```python
from build123d import *

# Parameters (mm, degrees)
F0_R      = 3.5
F1_DEPTH  = 4
F0_W      = 13
F0_H      = 4
F2_DEPTH  = 54
F3_R      = 5
F4_W      = 6.0393586755
F4_H      = 4
F5_DEPTH  = 5
F6_SIZE   = 3
F4_R      = 1.25
F7_DEPTH  = 49
F8_SIZE   = 1
F9_SIZE   = 1
F10_R     = 2.25
F11_DEPTH = 5
F12_R     = 2
F13_W     = 2
F13_H     = 22
F14_DEPTH = 5
F15_R     = 0.5


with BuildPart() as f1:
    # F0 (on Top) → F1 (new body)
    with BuildSketch(Plane.XY):
        with BuildLine():
            ThreePointArc((0, 5), (1.4644660941, 1.4644660941), (5, 0))
            Line((5, 0), (39, 0))
            Line((39, 0), (39, 10))
            Line((39, 10), (54, 10))
            Line((54, 10), (54, 0))
            Line((54, 0), (65, 0))
            Line((65, 0), (65, 10))
            Line((65, 10), (69, 10))
            Line((69, 10), (69, 0))
            Line((69, 0), (70, 0))
            ThreePointArc((70, 0), (73.5355339059, 1.4644660941), (75, 5))
            Line((75, 5), (75, 41))
            ThreePointArc((75, 41), (74.1213203436, 43.1213203436), (72, 44))
            Line((72, 44), (59, 44))
            Line((59, 44), (2.8562777384, 17.3555216386))
            ThreePointArc((2.8562777384, 17.3555216386), (0.7739728285, 15.5106003536), (0, 12.8383925874))
            Line((0, 12.8383925874), (0, 5))
        make_face()
        with Locations((14, 9)):
            Circle(F0_R, mode=Mode.SUBTRACT)
    extrude(amount=F1_DEPTH)

    # F0 (on Top) → F2 (join)
    with BuildSketch(Plane.XY):
        with Locations((65.5, 46)):
            Rectangle(F0_W, F0_H)
    extrude(amount=F2_DEPTH)

    # F3
    f3_edges = [f1.edges().sort_by_distance(p)[0] for p in [
        (72, 46, 54),
        (59, 46, 54),
    ]]
    fillet(f3_edges, radius=F3_R)

    # F4 (on face) → F5 (join)
    with BuildSketch(Plane.XY):
        Polygon((29.5861130485, 30.0408672094), (7.1886969879, 19.3925328106), (59, 19.3925328106), (59, 0), (65, 0), (65, 10), (65.0393586755, 10), (65.0393586755, 19.3925328106), (75, 19.3925328106), (75, 30.0408672094), (65.0393586755, 30.0408672094), (65.0393586755, 44), (59, 44), (59, 30.0408672094), align=None)
        with Locations((62.0196793377, 46)):
            Rectangle(F4_W, F4_H)
    extrude(amount=-F5_DEPTH)

    # F6 (call 1 of 4: OpenCascade refuses the feature's edges together)
    f6_edges = [f1.edges().sort_by_distance(p)[0] for p in [
        (62.019679, 48, -5),
        (75, 24.7167, -5),
        (70.019679, 30.040867, -5),
        (70.019679, 19.392533, -5),
        (65.039359, 39.020434, -5),
        (65.039359, 14.696266, -5),
    ]]
    chamfer(f6_edges, length=F6_SIZE)

    # F6#2 (call 2 of 4)
    f6_2_edges = [f1.edges().sort_by_distance(p)[0] for p in [
        (62, 0, -5),
    ]]
    chamfer(f6_2_edges, length=F6_SIZE)

    # F6#3 (call 3 of 4)
    f6_3_edges = [f1.edges().sort_by_distance(p)[0] for p in [
        (44.293057, 30.040867, -5),
    ]]
    chamfer(f6_3_edges, length=F6_SIZE)

    # F6#4 (call 4 of 4)
    f6_4_edges = [f1.edges().sort_by_distance(p)[0] for p in [
        (33.094348, 19.392533, -5),
    ]]
    chamfer(f6_4_edges, length=F6_SIZE)

    # F4 (on face) → F7 (join)
    with BuildSketch(Plane.XY):
        with Locations((72, 48)):
            Circle(F4_R)
    extrude(amount=F7_DEPTH)

    # F8
    f8_edges = [f1.edges().sort_by_distance(p)[0] for p in [
        (72.883883, 48.883883, 49),
    ]]
    chamfer(f8_edges, length=F8_SIZE)

    # F9
    f9_edges = [f1.edges().sort_by_distance(p)[0] for p in [
        (72.883883, 48.883883, 0),
    ]]
    chamfer(f9_edges, length=F9_SIZE)

    # F10 (on face) → F11 (cut)
    with BuildSketch(Plane(origin=(0, 48, 0), x_dir=(-1, 0, 0), z_dir=(0, 1, 0))):
        with Locations((-65.5, 11.5)):
            Circle(F10_R)
        with Locations((-65.5, 46.5)):
            Circle(F10_R)
    extrude(amount=-F11_DEPTH, mode=Mode.SUBTRACT)

    # F12
    f12_edges = [f1.edges().sort_by_distance(p)[0] for p in [
        (54, 10, 2),
        (54, 0, 2),
        (39, 10, 2),
        (39, 0, 2),
        (65, 0, 1),
        (69, 0, 2),
    ]]
    fillet(f12_edges, radius=F12_R)

    # F13 (on face) → F14 (cut)
    with BuildSketch(Plane(origin=(0, 48, 0), x_dir=(-1, 0, 0), z_dir=(0, 1, 0))):
        with Locations((-60, 29)):
            Rectangle(F13_W, F13_H)
    extrude(amount=-F14_DEPTH, mode=Mode.SUBTRACT)

    # F15
    f15_edges = [f1.edges().sort_by_distance(p)[0] for p in [
        (59, 46, 40),
        (59, 46, 18),
        (61, 46, 18),
        (61, 46, 40),
    ]]
    fillet(f15_edges, radius=F15_R)


solid = f1.part
```
Read the model definition and answer for the solid it produces. Units are mm, in the model's axes. A direction names the side the tool comes from. Coordinates: 2 decimals unless noted, no trailing zeros. Loops run counter-clockwise (first coordinate to the right, second up) from the corner with the lowest first, then second, coordinate; pieces in that order, holes last.
(1) A tool of negligible diameter and unlimited length cuts with its end or side. For faces 1 (the face through (69, 6, 2)), 2 (the face through (41.39, 28.56, -3.48)), 3 (the face through (65.039, 39, -1)), from which of +Z, -Z, +X, -X, +Y, -Y can it reach the whole face along a straight path? Write none if from no direction.
Solution:
face 1: +Z, -Z, -Y
face 2: -Z, -X, +Y
face 3: -Z, +X, +Y
(2) The part is cut by section C-C (x = 34). Determine the outline of the cut face in (y, z).
Solution:
outline: (0, 0) - (19.39, 0) - (19.39, -2) - (22.39, -5) - (27.04, -5) - (30.04, -2) - (30.04, 0) - (32.14, 0) - (32.14, 4) - (0, 4) - close
(3) Consider line 1 along Z through (x, y) = (65.5, 46); line 2 along Z through (x, y) = (65, 46); line 3 along Z through (x, y) = (14.5, 2). Determine where each line is inside the solid, lowest interval first.
Solution:
line 1: z = 0 to 9.25, 13.75 to 44.25, 48.75 to 54
line 2: z = -2.04 to 9.31, 13.69 to 44.31, 48.69 to 54
line 3: z = 0 to 4
(4) The part is cut by section B-B (y = 9). Determine the outline of the cut face in (x, z).
Solution:
outline: (0, 0) - (10.5, 0) - (10.5, 4) - (0, 4) - close; (17.5, 0) - (39.27, 0) - (39.27, 4) - (17.5, 4) - close; (53.73, 0) - (59, 0) - (59, -5) - (62.04, -5) - (65, -2.04) - (65, 4) - (53.73, 4) - close; (69, 0) - (75, 0) - (75, 4) - (69, 4) - close
(5) The part is cut by section A-A (z = 11.5). Determine the outline of the cut face in (x, y), and give its area (3 significant figures).
Solution:
outline: (59, 44) - (63.25, 44) - (63.25, 48) - (59, 48) - close; (67.75, 44) - (72, 44) - (72, 46.75) arc R1.25 ccw (long way) to (70.75, 48) - (67.75, 48) - close
area: 37.7 mm2
(6) The mould has two halves that part along Y. Classify faces 4 (the face through (46, 10, 2)), 5 (the face through (59, 11, -2)), 6 (the face through (70, 30.041, -1)), 7 (the face through (74.14, 43.1, 1.97)): released by +Y, released by -Y, zero draft, split by the parting line, or undercut.
Solution:
face 4: released by -Y
face 5: zero draft
face 6: released by +Y
face 7: undercut
(7) Flat-ended cylindrical pins translate along their axes: pin 1 Ø4 at (x, z) = (66, 30.5) entering from -Y; pin 2 Ø1.5 at (x, z) = (39.5, 4) entering from +Y; pin 3 Ø1.6 at (x, z) = (20.5, -1.5) entering from -Y; pin 4 Ø1.2 at (y, z) = (5.5, 2) entering from -X. Find the tip coordinate at first contact, or state that the pin passes through.
Solution:
pin 1: stops at y = 44
pin 2: stops at y = 35.1
pin 3: stops at y = 19.39
pin 4: stops at x = 0
